from build123d import *

# Parameters (mm, degrees)
SKETCH1_W           = 12.05
SKETCH1_H           = 22.45
BOSS_EXTRUDE2_DEPTH = 20
SKETCH6_W           = 35.864128229
SKETCH6_H           = 30.191250037
BOSS_EXTRUDE3_DEPTH = 20
SKETCH7_W           = 35
SKETCH7_H           = 32
CUT_EXTRUDE3_DEPTH  = 13


with BuildPart() as part:
    # Sketch1 → Boss-Extrude2 (new body)
    with BuildSketch(Plane(origin=(0, 0, 0), x_dir=(1, 0, 0), z_dir=(0, 1, 0))):
        Polygon((-39.417705009, -78.511923184), (-39.417705009, -39.511923184), (-18.417705009, -39.511923184), (2.582294991, -39.511923184), (2.582294991, -78.511923184), (2.582294991, -106.961923184), (-18.417705009, -106.961923184), (-39.417705009, -106.961923184), align=None)
        with Locations((-27.392705009, -89.736923184)):
            Rectangle(SKETCH1_W, SKETCH1_H, mode=Mode.SUBTRACT)
        Polygon((-33.417705009, -70.511923184), (-33.417705009, -45.511923184), (-18.417705009, -45.511923184), (-3.417705009, -45.511923184), (-3.417705009, -70.511923184), align=None, mode=Mode.SUBTRACT)
        with Locations((-9.442705009, -89.736923184)):
            Rectangle(SKETCH1_W, SKETCH1_H, mode=Mode.SUBTRACT)
    extrude(amount=BOSS_EXTRUDE2_DEPTH)

    # Sketch6 → Boss-Extrude3 (add)
    with BuildSketch(Plane(origin=(0, 20, 0), x_dir=(1, 0, 0), z_dir=(0, 1, 0))):
        with Locations((-18.754231682, -88.861375831)):
            Rectangle(SKETCH6_W, SKETCH6_H)
    extrude(amount=-BOSS_EXTRUDE3_DEPTH)

    # Sketch7 → Cut-Extrude3 (cut)
    with BuildSketch(Plane(origin=(0, 20, 0), x_dir=(1, 0, 0), z_dir=(0, 1, 0))):
        with Locations((-18.421350721, -88.672765983)):
            Rectangle(SKETCH7_W, SKETCH7_H)
    extrude(amount=-CUT_EXTRUDE3_DEPTH, mode=Mode.SUBTRACT)


solid = part.part
Part model, mm, in its own coordinate system. A direction names the side the tool comes from. Coordinates: 2 decimals unless noted, no trailing zeros. Order: outer loops, then holes, each group sorted by start corner. A loop starts at its lowest first (then second) coordinate and runs counter-clockwise, first axis right, second up. Notation, with made-up numbers: M 43,63 L 67,63 A26 ccw 67,82 Z; hole C 35.25,56.25 d10. An arc over 180 degrees is marked long. One line per question, with ' | ' between items.
Q1. Slice it at B-B (y = 11.75). Give the cut face in (x, z), and give its area (3 significant figures).
A:
outline: M -39.42,39.51 L 2.58,39.51 L 2.58,106.96 L -39.42,106.96 Z; hole M -35.92,72.67 L -0.92,72.67 L -0.92,104.67 L -35.92,104.67 Z; hole M -33.42,45.51 L -3.42,45.51 L -3.42,70.51 L -33.42,70.51 Z | area: 963 mm^2
Q2. Slice it at C-C (z = 47). Give the cut face in (x, y).
A:
outline: M -39.42,0 L -33.42,0 L -33.42,20 L -39.42,20 Z; M -3.42,0 L 2.58,0 L 2.58,20 L -3.42,20 Z
Q3. Pin check, flat tip, straight feed: P1, Ø1, axis at x = -12.5, z = 97, coming from the +Y side. Stop position of the tip, or through.
A:
P1: stops at y = 7
Q4. Slice it at A-A (x = -25). Give the cut face in (y, z), and give its area (3 significant figures).
A:
outline: M 0,39.51 L 20,39.51 L 20,45.51 L 0,45.51 Z; M 0,70.51 L 20,70.51 L 20,72.67 L 7,72.67 L 7,104.67 L 20,104.67 L 20,106.96 L 0,106.96 Z | area: 433 mm^2
Q5. 3-axis set-ups, long thin cutter, end or side, ignore diameter. For faces 4 (the face through (-19, 10, 106.962)), 5 (the face through (-19, 14, 72.673)), 6 (the face through (-18, 10, 70.512)): which of +Z, -Z, +X, -X, +Y, -Y reach the whole face in a straight line?
A:
face 4: +Z, +X, -X, +Y, -Y | face 5: +Y | face 6: +Y, -Y
Q6. Slice it at D-D (z = 89.5). Give the cut face in (x, y).
A:
outline: M -39.42,0 L 2.58,0 L 2.58,20 L -0.92,20 L -0.92,7 L -35.92,7 L -35.92,20 L -39.42,20 Z
Q7. Two-plate mould, pull along Z, no slides. Class faces 1 (the face through (-18, 10, 39.512)), 2 (the face through (-3.418, 10, 58)), 3 (the face through (-18, 0, 80)): +Z half, -Z half, draft (parallel to the pull), parting line (faces both ways), or undercut.
A:
face 1: -Z half | face 2: undercut | face 3: draft
Q8. Drill centre lines: line 1 (Z direction, x = -31.5, y = 7.75); line 2 (X direction, y = 18.75, z = 49.5); line 3 (Z direction, x = -20, y = 6). Where is each one in solid material? Low to high.
A:
line 1: z = 39.51 to 45.51, 70.51 to 72.67, 104.67 to 106.96 | line 2: x = -39.42 to -33.42, -3.42 to 2.58 | line 3: z = 39.51 to 45.51, 70.51 to 106.96
